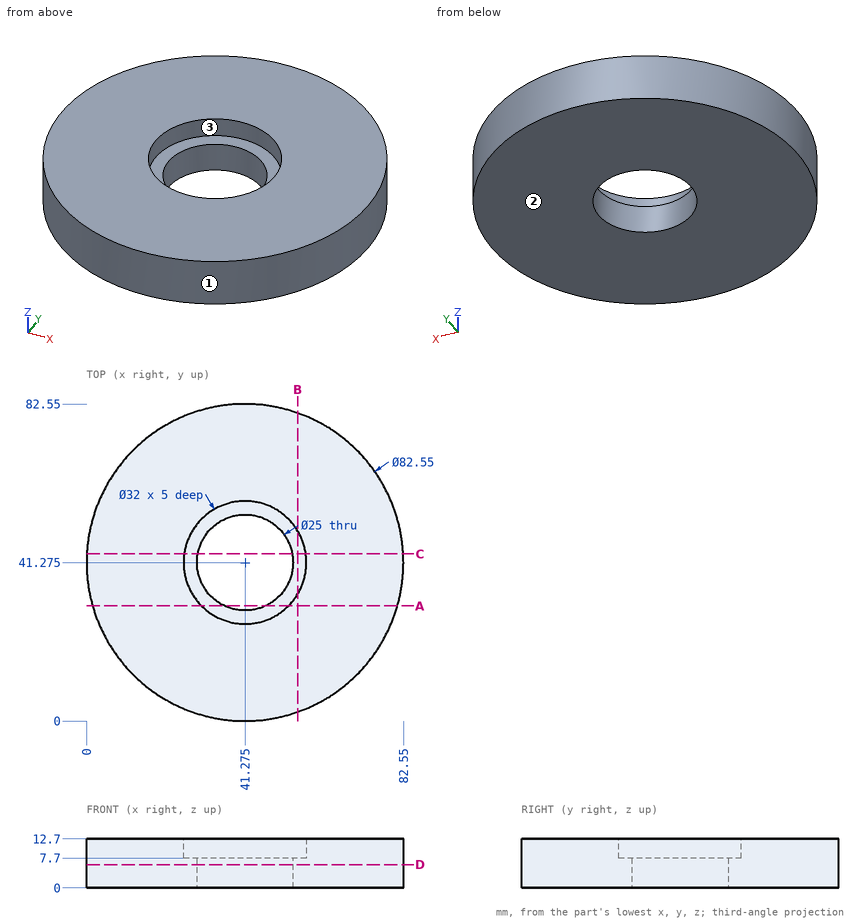
Design review of the part shown in the three views and the two pictorial views. Dimensions are in mm from the part's minimum x, y and z. Coordinates: 2 decimals unless noted, no trailing zeros. Write each loop counter-clockwise with the first axis right and the second up, starting at its lowest first coordinate (ties: lowest second). Pieces come first, ordered by that corner, then holes.
1) We need section B-B on x = 55. State the section outline as (y, z) points, then the cut area to 3 significant figures.
2) To check wall thickness, follow probe 1 along X at (y, z) = (34.5, 10.25); probe 2 along Y at (x, z) = (39, 6.25); probe 3 along X at (y, z) = (39.5, 7). State the ranges of each line that lie inside material, in increasing order.
3) We need section A-A on y = 30. State the section outline as (x, z) points.
4) Clearance check with flat-ended pins moving along their axes: pin 1 Ø1.5 at (y, z) = (68, 6) entering from -X; pin 2 Ø2 at (y, z) = (29, 2) entering from -X; pin 3 Ø4 at (x, z) = (35, 5) entering from +Y. State where each tip first meets the part, or that it passes through.
5) We need section C-C on y = 43.5. State the section outline as (x, z) points, then the cut area to 3 significant figures.
6) We need section D-D on z = 6. State the section outline as (x, y) points (3 decimals), then the cut area to 3 significant figures.
7) The part is to be moulded in two halves that separate along Y. For the marked faces 1, 2 and 3, say which applies: pulls with the +Y half, pulls with the -Y half, needs draft (parallel to the pull), parting line crosses it, or undercut.
Answer list:
1. outline: (2.35, 0) - (80.2, 0) - (80.2, 12.7) - (49.5, 12.7) - (49.5, 7.7) - (33.05, 7.7) - (33.05, 12.7) - (2.35, 12.7) - close
1. area: 906 mm2
2. probe 1: x = 0.56 to 26.78, 55.77 to 81.99
2. probe 2: y = 0.06 to 28.98, 53.57 to 82.49
2. probe 3: x = 0.04 to 28.9, 53.65 to 82.51
3. outline: (1.57, 0) - (35.88, 0) - (35.88, 7.7) - (29.92, 7.7) - (29.92, 12.7) - (1.57, 12.7) - close; (46.67, 0) - (80.98, 0) - (80.98, 12.7) - (52.63, 12.7) - (52.63, 7.7) - (46.67, 7.7) - close
4. pin 1: stops at x = 9.2
4. pin 2: stops at x = 1.57
4. pin 3: stops at y = 82.33
5. outline: (0.06, 0) - (28.97, 0) - (28.97, 7.7) - (25.43, 7.7) - (25.43, 12.7) - (0.06, 12.7) - close; (53.58, 0) - (82.49, 0) - (82.49, 12.7) - (57.12, 12.7) - (57.12, 7.7) - (53.58, 7.7) - close
5. area: 699 mm2
6. outline: circle Ø82.55 at (41.275, 41.275); hole circle Ø25 at (41.275, 41.275)
6. area: 4,860 mm2
7. face 1: parting line crosses it
7. face 2: needs draft
7. face 3: undercut
